Here's how the part is built. I have some questions about the finished solid (model axes, mm). Face numbers are marked on the shaded views. A direction names the side the tool comes from. Give positions to 0.01 mm unless a question says otherwise; leave off trailing zeros. One line per item, written item: value. Start each with the question number.
1) Please list where these lines run through material, in increasing order: L1, parallel to X at y = 95, z = 6; L2, parallel to X at y = 10, z = -26; L3, parallel to Z at x = 16.75, y = 52.5. Write a range as [from, to].
2) On a 3-axis mill with a long thin cutter (end or side, diameter ignored), from which of +Z, -Z, +X, -X, +Y, -Y can I reach the whole of each face in a straight line? I mean the marked faces 1, 2 and 3. Say none if no direction works.
3) I'm going to push flat-ended pins straight in: P1, Ø4, axis at x = 8, y = 34.5, coming from the -Z side; P2, Ø4, axis at x = 8, y = 49.5, coming from the -Z side; P3, Ø5, axis at x = 6.5, y = 41.5, coming from the -Z side. Where does each tip first touch, or does it pass through?
4) We'd pull the mould along Z, two halves only. Please class the marked faces 4, 5 and 6: +Z half, -Z half, draft (parallel to the pull), parting line (faces both ways), or undercut.
5) Imagine slicing it at A-A on x = 11.43. Count the separate pieces of the cut face and the enclosed holes in it, plus the area to 3 significant figures.
from build123d import *

# Parameters (mm, degrees)
BOSS_EXTRUDE1_DEPTH = 22.86
SKETCH2_R           = 4.7625
CUT_EXTRUDE1_DEPTH  = 70.0372
SKETCH3_R           = 9.4615
CUT_EXTRUDE2_DEPTH  = 23.86
FILLET1_R           = 3.175


with BuildPart() as part:
    # Sketch1 → Boss-Extrude1 (new body)
    with BuildSketch(Plane(origin=(0, 0, 0), x_dir=(0, 0, -1), z_dir=(1, 0, 0))):
        with BuildLine():
            Line((43.6372, 0), (43.6372, 31.75))
            ThreePointArc((43.6372, 31.75), (46.914198612, 50.033148662), (56.3372, 66.04))
            Line((56.3372, 66.04), (56.3372, 106.68))
            Line((56.3372, 106.68), (34.5186, 106.68))
            Line((34.5186, 106.68), (34.5186, 81.28))
            Line((34.5186, 81.28), (9.1186, 81.28))
            Line((9.1186, 81.28), (9.1186, 106.68))
            Line((9.1186, 106.68), (-12.7, 106.68))
            Line((-12.7, 106.68), (-12.7, 66.04))
            ThreePointArc((-12.7, 66.04), (-3.276998612, 50.033148662), (0, 31.75))
            Line((0, 31.75), (0, 0))
            Line((0, 0), (43.6372, 0))
        make_face()
    extrude(amount=BOSS_EXTRUDE1_DEPTH)

    # Sketch2 → Cut-Extrude1 (cut, through all)
    with BuildSketch(Plane.XY.offset(12.7)):
        with Locations((11.43, 95.25)):
            Circle(SKETCH2_R)
        with Locations((11.43, 11.43)):
            Circle(SKETCH2_R)
    extrude(amount=-CUT_EXTRUDE1_DEPTH, mode=Mode.SUBTRACT)

    # Sketch3 → Cut-Extrude2 (cut, through all)
    with BuildSketch(Plane(origin=(22.86, 0, 0), x_dir=(0, 0, -1), z_dir=(1, 0, 0))):
        with Locations((21.8186, 53.34)):
            Circle(SKETCH3_R)
    extrude(amount=-CUT_EXTRUDE2_DEPTH, mode=Mode.SUBTRACT)

    # Fillet1
    fillet1_edges = [part.edges().sort_by_distance(p)[0] for p in [
        (22.86, 50.033148662, -46.914198612),
        (0, 15.875, 0),
        (0, 50.033148662, 3.276998612),
        (0, 86.36, 12.7),
        (0, 106.68, 1.7907),
        (0, 93.98, -9.1186),
        (0, 81.28, -21.8186),
        (22.86, 86.36, -56.3372),
        (0, 93.98, -34.5186),
        (0, 106.68, -45.4279),
        (0, 86.36, -56.3372),
        (0, 50.033148662, -46.914198612),
        (0, 15.875, -43.6372),
        (0, 0, -21.8186),
        (22.86, 106.68, -45.4279),
        (22.86, 93.98, -34.5186),
        (11.43, 0, 0),
        (11.43, 106.68, 12.7),
        (11.43, 106.68, -9.1186),
        (11.43, 106.68, -34.5186),
        (11.43, 106.68, -56.3372),
        (11.43, 0, -43.6372),
        (22.86, 81.28, -21.8186),
        (22.86, 93.98, -9.1186),
        (22.86, 106.68, 1.7907),
        (22.86, 86.36, 12.7),
        (22.86, 50.033148662, 3.276998612),
        (22.86, 15.875, 0),
        (22.86, 0, -21.8186),
        (22.86, 15.875, -43.6372),
    ]]
    fillet(fillet1_edges, radius=FILLET1_R)


solid = part.part
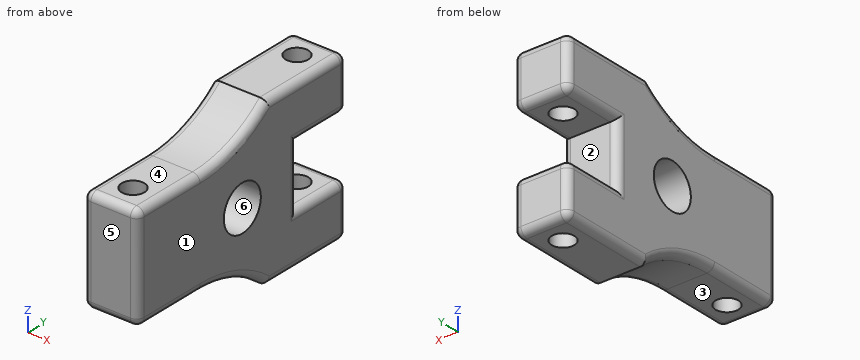
Numbers:
1. L1: [0, 6.67], [16.19, 22.86]
1. L2: [0, 6.89], [15.97, 22.86]
1. L3: [-47.9, -31.24], [-12.39, 4.26]
2. face 1: +Z, -Z, +X, +Y, -Y
2. face 2: +X, -X, +Y
2. face 3: -Z, +X, -X, -Y
3. P1: z = -43.85
3. P2: z = -47.48
3. P3: z = -45.08
4. face 4: +Z half
4. face 5: draft
4. face 6: undercut
5. separate pieces: 4
5. enclosed holes: 1
5. area: 4,190 mm^2
